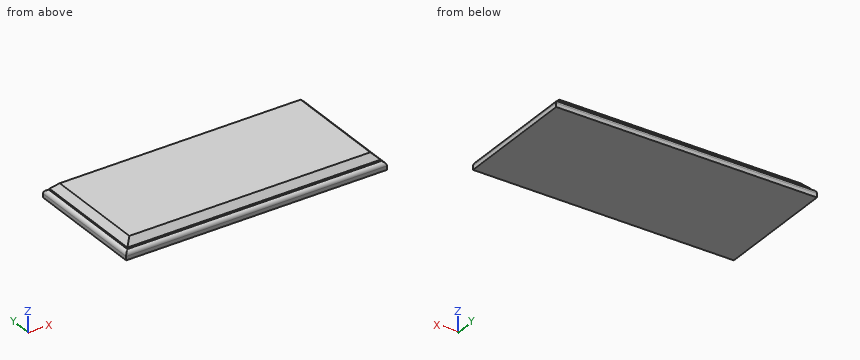
```python
from build123d import *

# Parameters (mm, degrees)
F0_W     = 215.9
F0_H     = 101.6
F1_DEPTH = 6.35
F2_R     = 3.175
F3_DEPTH = 6.35
F4_SIZE  = 5.08


with BuildPart() as f1:
    # F0 (on Top) → F1 (new body)
    with BuildSketch(Plane.XY):
        with Locations((-16.8649114484, -0.8375608661)):
            Rectangle(F0_W, F0_H)
    extrude(amount=F1_DEPTH)

    # F2
    f2_edges = [f1.edges().sort_by_distance(p)[0] for p in [
        (-16.864911, -51.637561, 6.35),
        (91.085089, -0.837561, 6.35),
        (-16.864911, 49.962439, 6.35),
        (-124.814911, -0.837561, 6.35),
    ]]
    fillet(f2_edges, radius=F2_R)

    # F3 (add): a face of the model
    f3_faces = [f1.faces().sort_by_distance(p)[0] for p in [
        (-16.8649114484, -0.8375608661, 6.35),
    ]]
    extrude(f3_faces, amount=F3_DEPTH)

    # F4
    f4_edges = [f1.edges().sort_by_distance(p)[0] for p in [
        (-16.864911, -48.462561, 12.7),
        (-121.639911, -0.837561, 12.7),
        (87.910089, -0.837561, 12.7),
        (-16.864911, 46.787439, 12.7),
    ]]
    chamfer(f4_edges, length=F4_SIZE)


solid = f1.part
```
Part model, mm, in its own coordinate system. Round coordinates to 2 decimals unless told otherwise and drop trailing zeros. Loops run counter-clockwise (first coordinate to the right, second up) from the corner with the lowest first, then second, coordinate; pieces in that order, holes last.
Item 1: Drop flat-ended pins along their axis: P1, Ø1, axis at x = -67, z = 7, coming from the +Y side; P2, Ø0.6, axis at x = -31.5, z = 7, coming from the -Y side; P3, Ø0.6, axis at y = -11, z = 7, coming from the +X side. Give the stop position or say it passes through.
Item 2: Cut at B-B, the plane x = -86.5. Give the cut face in (y, z) (3 decimals).
Item 3: Cut at A-A, the plane y = -10. Give the cut face in (x, z) (3 decimals).
Item 4: Drill centre lines: line 1 (X direction, y = 25, z = 7.5); line 2 (Y direction, x = -57.5, z = 7.5); line 3 (X direction, y = -17, z = 11.5). Where is each one in solid material? Low to high.
A:
1. P1: stops at y = 46.79
1. P2: stops at y = -48.46
1. P3: stops at x = 87.91
2. outline: (-51.638, 0) - (49.962, 0) - (49.962, 3.175) arc R3.175 ccw to (46.787, 6.35) - (46.787, 7.62) - (41.707, 12.7) - (-43.383, 12.7) - (-48.463, 7.62) - (-48.463, 6.35) arc R3.175 ccw to (-51.638, 3.175) - close
3. outline: (-124.815, 0) - (91.085, 0) - (91.085, 3.175) arc R3.175 ccw to (87.91, 6.35) - (87.91, 7.62) - (82.83, 12.7) - (-116.56, 12.7) - (-121.64, 7.62) - (-121.64, 6.35) arc R3.175 ccw to (-124.815, 3.175) - close
4. line 1: x = -121.64 to 87.91
4. line 2: y = -48.46 to 46.79
4. line 3: x = -117.76 to 84.03
